Geometry check sheet. Reference: the model listing, model coordinates, mm. Coordinates: 2 decimals unless noted, no trailing zeros. Write each loop counter-clockwise with the first axis right and the second up, starting at its lowest first coordinate (ties: lowest second). Pieces come first, ordered by that corner, then holes. Notation, with made-up numbers: (79.25, -35.5) -> (91.25, -35.5) arc R14 ccw to (91.25, -26.5) -> close; hole circle Ø1 at (-1, 7.5). An arc over 180 degrees is marked (long way). Use a Markdown table: item, result.
```python
from build123d import *

# Parameters (mm, degrees)
SKETCH1_R           = 40
SKETCH1_R_2         = 1.5
SKETCH1_R_3         = 37
BOSS_EXTRUDE1_DEPTH = 8
SKETCH3_R           = 40
CUT_EXTRUDE1_DEPTH  = 4
SKETCH4_R           = 3
SKETCH4_R_2         = 1.5
CUT_EXTRUDE2_DEPTH  = 4


with BuildPart() as part:
    # Sketch1 → Boss-Extrude1 (new body)
    # profile 1 of 2: a face of its own
    with BuildSketch(Plane.XY):
        with BuildLine():
            Line((51.719126793, -47), (55, 0))
            ThreePointArc((55, 0), (0, 55), (-55, 0))
            Line((-55, 0), (-51.719126793, -47))
            Line((-51.719126793, -47), (-51.719126793, -57))
            Line((-51.719126793, -57), (-41.694792144, -57))
            Line((-41.694792144, -57), (41.694792144, -57))
            Line((41.694792144, -57), (51.719126793, -57))
            Line((51.719126793, -57), (51.719126793, -47))
        make_face()
        Circle(SKETCH1_R, mode=Mode.SUBTRACT)
        with Locations((46.719126793, -52)):
            Circle(SKETCH1_R_2, mode=Mode.SUBTRACT)
        with Locations((48.371701184, -23.151818224)):
            Circle(SKETCH1_R_2, mode=Mode.SUBTRACT)
        with Locations((49.240387651, 8.682408883)):
            Circle(SKETCH1_R_2, mode=Mode.SUBTRACT)
        with Locations((32.139380484, 38.302222156)):
            Circle(SKETCH1_R_2, mode=Mode.SUBTRACT)
        with Locations((0, 50)):
            Circle(SKETCH1_R_2, mode=Mode.SUBTRACT)
        with Locations((-32.139380484, 38.302222156)):
            Circle(SKETCH1_R_2, mode=Mode.SUBTRACT)
        with Locations((-49.240387651, 8.682408883)):
            Circle(SKETCH1_R_2, mode=Mode.SUBTRACT)
        with Locations((-48.371701184, -23.151818224)):
            Circle(SKETCH1_R_2, mode=Mode.SUBTRACT)
        with Locations((-46.719126793, -52)):
            Circle(SKETCH1_R_2, mode=Mode.SUBTRACT)
    # profile 2 of 2: a face of its own
    with BuildSketch(Plane.XY):
        Circle(SKETCH1_R)
        Circle(SKETCH1_R_3, mode=Mode.SUBTRACT)
    extrude(amount=BOSS_EXTRUDE1_DEPTH)

    # Sketch3 → Cut-Extrude1 (cut)
    with BuildSketch(Plane.XY.offset(8)):
        Circle(SKETCH3_R)
    extrude(amount=-CUT_EXTRUDE1_DEPTH, mode=Mode.SUBTRACT)

    # Sketch4 → Cut-Extrude2 (cut)
    # profile 1 of 9: a face of its own
    with BuildSketch(Plane(origin=(0, 0, 0), x_dir=(-1, 0, 0), z_dir=(0, 0, -1))):
        with Locations((-46.719126793, -52)):
            Circle(SKETCH4_R)
        with Locations((-46.719126793, -52)):
            Circle(SKETCH4_R_2, mode=Mode.SUBTRACT)
    # profile 2 of 9: a face of its own
    with BuildSketch(Plane(origin=(0, 0, 0), x_dir=(-1, 0, 0), z_dir=(0, 0, -1))):
        with Locations((-48.371701184, -23.151818224)):
            Circle(SKETCH4_R)
        with Locations((-48.371701184, -23.151818224)):
            Circle(SKETCH4_R_2, mode=Mode.SUBTRACT)
    # profile 3 of 9: a face of its own
    with BuildSketch(Plane(origin=(0, 0, 0), x_dir=(-1, 0, 0), z_dir=(0, 0, -1))):
        with Locations((-49.240387651, 8.682408883)):
            Circle(SKETCH4_R)
        with Locations((-49.240387651, 8.682408883)):
            Circle(SKETCH4_R_2, mode=Mode.SUBTRACT)
    # profile 4 of 9: a face of its own
    with BuildSketch(Plane(origin=(0, 0, 0), x_dir=(-1, 0, 0), z_dir=(0, 0, -1))):
        with Locations((-32.139380484, 38.302222156)):
            Circle(SKETCH4_R)
        with Locations((-32.139380484, 38.302222156)):
            Circle(SKETCH4_R_2, mode=Mode.SUBTRACT)
    # profile 5 of 9: a face of its own
    with BuildSketch(Plane(origin=(0, 0, 0), x_dir=(-1, 0, 0), z_dir=(0, 0, -1))):
        with Locations((0, 50)):
            Circle(SKETCH4_R)
        with Locations((0, 50)):
            Circle(SKETCH4_R_2, mode=Mode.SUBTRACT)
    # profile 6 of 9: a face of its own
    with BuildSketch(Plane(origin=(0, 0, 0), x_dir=(-1, 0, 0), z_dir=(0, 0, -1))):
        with Locations((32.139380484, 38.302222156)):
            Circle(SKETCH4_R)
        with Locations((32.139380484, 38.302222156)):
            Circle(SKETCH4_R_2, mode=Mode.SUBTRACT)
    # profile 7 of 9: a face of its own
    with BuildSketch(Plane(origin=(0, 0, 0), x_dir=(-1, 0, 0), z_dir=(0, 0, -1))):
        with Locations((49.240387651, 8.682408883)):
            Circle(SKETCH4_R)
        with Locations((49.240387651, 8.682408883)):
            Circle(SKETCH4_R_2, mode=Mode.SUBTRACT)
    # profile 8 of 9: a face of its own
    with BuildSketch(Plane(origin=(0, 0, 0), x_dir=(-1, 0, 0), z_dir=(0, 0, -1))):
        with Locations((48.371701184, -23.151818224)):
            Circle(SKETCH4_R)
        with Locations((48.371701184, -23.151818224)):
            Circle(SKETCH4_R_2, mode=Mode.SUBTRACT)
    # profile 9 of 9: a face of its own
    with BuildSketch(Plane(origin=(0, 0, 0), x_dir=(-1, 0, 0), z_dir=(0, 0, -1))):
        with Locations((46.719126793, -52)):
            Circle(SKETCH4_R)
        with Locations((46.719126793, -52)):
            Circle(SKETCH4_R_2, mode=Mode.SUBTRACT)
    extrude(amount=-CUT_EXTRUDE2_DEPTH, mode=Mode.SUBTRACT)


solid = part.part
```
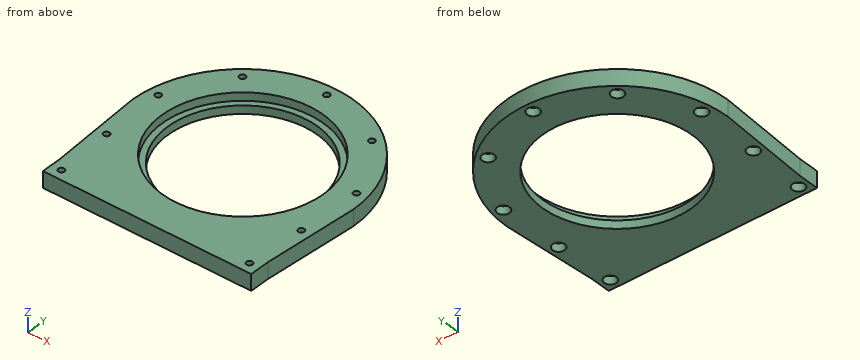
Item 1: Section check C-C on y = 30. Record the boundary of the cut face in (x, z).
Answer block:
| item | result |
|---|---|
| outline | (-46.1, 0) -> (-21.66, 0) -> (-21.66, 4) -> (-26.46, 4) -> (-26.46, 8) -> (-46.1, 8) -> close; (21.66, 0) -> (46.1, 0) -> (46.1, 8) -> (26.46, 8) -> (26.46, 4) -> (21.66, 4) -> close |
Item 2: Depth check by flat-ended pin: P1, Ø4, axis at x = -36.5, y = 9, coming from the +Z side; P2, Ø1.8, axis at x = 46.72, y = -52, coming from the -Z side; P3, Ø1.8, axis at x = 47.5, y = -51, coming from the -Z side; P4, Ø4, axis at y = 4, z = 6, coming from the -X side. Enter the tip coordinate at first touch or a pass-through.
Answer block:
| item | result |
|---|---|
| P1 | stops at z = 4 |
| P2 | passes through |
| P3 | stops at z = 4 |
| P4 | stops at x = -54.96 |
Item 3: Thickness scan on L1, parallel to Y at x = 0, z = 6.3; L2, parallel to X at y = 1.5, z = 7; L3, parallel to Y at x = -32, z = 0.75. Record the ranges inside material, lowest first. Write a range as [from, to].
Answer block:
| item | result |
|---|---|
| L1 | y = [-57, -40], [40, 48.5], [51.5, 55] |
| L2 | x = [-54.98, -39.97], [39.97, 54.98] |
| L3 | y = [-57, -18.57], [18.57, 35.31], [41.3, 44.73] |
Item 4: Section check A-A on x = 0. Record the boundary of the cut face in (y, z), then the cut area to 3 significant figures.
Answer block:
| item | result |
|---|---|
| outline | (-57, 0) -> (-37, 0) -> (-37, 4) -> (-40, 4) -> (-40, 8) -> (-57, 8) -> close; (37, 0) -> (47, 0) -> (47, 4) -> (48.5, 4) -> (48.5, 8) -> (40, 8) -> (40, 4) -> (37, 4) -> close; (51.5, 4) -> (53, 4) -> (53, 0) -> (55, 0) -> (55, 8) -> (51.5, 8) -> close |
| area | 244 mm^2 |
Item 5: Section check D-D on z = 1.75. Count the separate pieces of the cut face and the enclosed holes in it, then the cut area to 3 significant figures.
Answer block:
| item | result |
|---|---|
| separate pieces | 1 |
| enclosed holes | 10 |
| area | 6,250 mm^2 |
Item 6: Section check B-B on y = -52. Record the boundary of the cut face in (x, z), then the cut area to 3 significant figures.
Answer block:
| item | result |
|---|---|
| outline | (-51.72, 0) -> (-49.72, 0) -> (-49.72, 4) -> (-48.22, 4) -> (-48.22, 8) -> (-51.72, 8) -> close; (-45.22, 4) -> (-43.72, 4) -> (-43.72, 0) -> (43.72, 0) -> (43.72, 4) -> (45.22, 4) -> (45.22, 8) -> (-45.22, 8) -> close; (48.22, 4) -> (49.72, 4) -> (49.72, 0) -> (51.72, 0) -> (51.72, 8) -> (48.22, 8) -> close |
| area | 756 mm^2 |
